Geometry check sheet. Reference: the model listing, model coordinates, mm. A direction names the side the tool comes from. Coordinates: 2 decimals unless noted, no trailing zeros. Write each loop counter-clockwise with the first axis right and the second up, starting at its lowest first coordinate (ties: lowest second). Pieces come first, ordered by that corner, then holes. Notation, with made-up numbers: (76.5, 6.5) -> (88.5, 6.5) arc R29 cw to (88.5, 29.5) -> close; hole circle Ø9 at (19, 48.25). An arc over 180 degrees is marked (long way). One line per question, with ' | ' between items.
```python
from build123d import *

# Parameters (mm, degrees)
F0_W          = 50
F0_H          = 50
F0_W_2        = 40
F0_H_2        = 40
F1_DEPTH      = 202
F3_DEPTH      = 25.001
F3_DEPTH_BACK = 25.001


with BuildPart() as f1:
    # F0 (on Front) → F1 (new body, symmetric)
    with BuildSketch(Plane.XZ):
        Rectangle(F0_W, F0_H)
        Rectangle(F0_W_2, F0_H_2, mode=Mode.SUBTRACT)
    extrude(amount=F1_DEPTH, both=True)

    # F2 (on Top) → F3 (cut, two sides)
    with BuildSketch(Plane.XY) as f3_sk:
        Polygon((-25, 184), (25, 202), (-25, 202), align=None)
        Polygon((-25, -202), (25, -202), (-25, -184), align=None)
    extrude(amount=-F3_DEPTH, mode=Mode.SUBTRACT)
    extrude(f3_sk.sketch, amount=F3_DEPTH_BACK, mode=Mode.SUBTRACT)


solid = f1.part
```
(1) Tool access check on faces 5 (the face through (0, -3, -20)), 6 (the face through (0, 193, 22)). Record the directions out of +Z, -Z, +X, -X, +Y, -Y that give a thin tool (end or side, any length) a straight path to the whole face; none if there is none.
Answers below:
face 5: +Y, -Y | face 6: +Z, -Z, -X, +Y
(2) Cross-section at B-B (x = -16). Record the cut outline in (y, z).
Answers below:
outline: (-187.24, -25) -> (187.24, -25) -> (187.24, -20) -> (-187.24, -20) -> close; (-187.24, 20) -> (187.24, 20) -> (187.24, 25) -> (-187.24, 25) -> close
(3) Depth check by flat-ended pin: P1, Ø8, axis at x = 14, z = 20, coming from the -Y side. Enter the tip coordinate at first touch or a pass-through.
Answers below:
P1: stops at y = -199.48
(4) Material ranges on line 1 (Z direction, x = -19, y = -3.5); line 2 (Y direction, x = 21, z = -5), recorded low to high.
Answers below:
line 1: z = -25 to -20, 20 to 25 | line 2: y = -200.56 to 200.56
(5) Draft check along X on faces 1 (the face through (-25, -3, 0)), 2 (the face through (20, -3, 0)), 3 (the face through (0, -3, 25)), 4 (the face through (0, -3, 20)). Enter one of: pulls with the +X half, pulls with the -X half, needs draft (parallel to the pull), parting line crosses it, or undercut.
Answers below:
face 1: pulls with the -X half | face 2: undercut | face 3: needs draft | face 4: undercut
(6) Cross-section at A-A (z = 11). Record the cut outline in (x, y).
Answers below:
outline: (-25, -184) -> (-20, -185.8) -> (-20, 185.8) -> (-25, 184) -> close; (20, -200.2) -> (25, -202) -> (25, 202) -> (20, 200.2) -> close
(7) Cross-section at C-C (y = 160). Record the cut outline in (x, z), plus the area to 3 significant figures.
Answers below:
outline: (-25, -25) -> (25, -25) -> (25, 25) -> (-25, 25) -> close; hole (-20, -20) -> (20, -20) -> (20, 20) -> (-20, 20) -> close | area: 900 mm²
